Geometry: final body of the model. Coordinates: model frame, mm. Face numbers are marked on the shaded views. A direction names the side the tool comes from. Round coordinates to 2 decimals unless told otherwise and drop trailing zeros. Write each loop counter-clockwise with the first axis right and the second up, starting at its lowest first coordinate (ties: lowest second). Pieces come first, ordered by that corner, then holes.
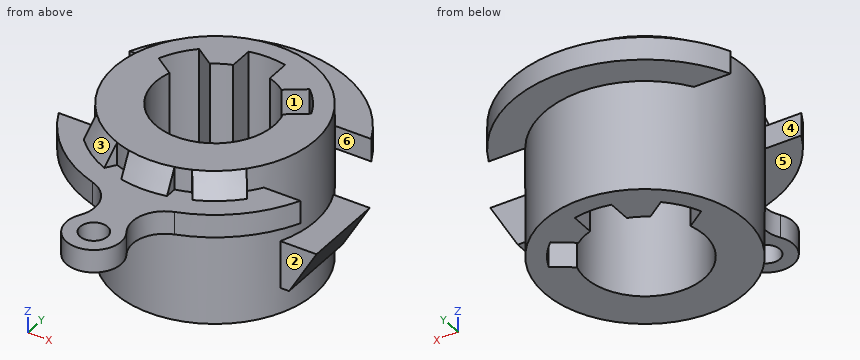
from build123d import *

# Parameters (mm, degrees)
F0_R      = 44
F1_DEPTH  = 34
F3_R      = 6
F4_DEPTH  = 10
F5_W      = 12.3737903833
F5_H      = 20.7846096908
F6_DEPTH  = 18
F4_FACE_R = 6
F8_DEPTH  = 10
F12_DEPTH = 107.2


with BuildPart() as f1:
    # F0 (on Top) → F1 (new body, symmetric)
    with BuildSketch(Plane.XY):
        Circle(F0_R)
        with BuildLine():
            ThreePointArc((-15.6760909215, 20.742713743), (-12.0054639441, 23.0622816626), (-8, 24.7386337537))
            Line((-8, 24.7386337537), (-8, 35.0998575496))
            ThreePointArc((-8, 35.0998575496), (0, 36), (8, 35.0998575496))
            Line((8, 35.0998575496), (8, 24.7386337537))
            ThreePointArc((8, 24.7386337537), (12.0054639441, 23.0622816626), (15.6760909215, 20.742713743))
            Line((15.6760909215, 20.742713743), (24.1635085752, 26.685667564))
            ThreePointArc((24.1635085752, 26.685667564), (29.4894735944, 20.6487517086), (33.3407315568, 13.5792348554))
            Line((33.3407315568, 13.5792348554), (24.8533139031, 7.6362810343))
            ThreePointArc((24.8533139031, 7.6362810343), (0, -26), (-24.8533139031, 7.6362810343))
            Line((-24.8533139031, 7.6362810343), (-33.3407315568, 13.5792348554))
            ThreePointArc((-33.3407315568, 13.5792348554), (-29.4894735944, 20.6487517086), (-24.1635085752, 26.685667564))
            Line((-24.1635085752, 26.685667564), (-15.6760909215, 20.742713743))
        make_face(mode=Mode.SUBTRACT)
    extrude(amount=F1_DEPTH, both=True)

    # F3 (on offset) → F4 (join)
    with BuildSketch(Plane.XY.offset(24)):
        with BuildLine():
            Line((-36.8781778292, -24), (-52.8015151298, -24))
            ThreePointArc((-52.8015151298, -24), (-38.6311115614, -43.2624227191), (-17.8938638331, -55.1707317073))
            ThreePointArc((-17.8938638331, -55.1707317073), (-9.0876412514, -63.6171726174), (-10.252187236, -75.7636022514))
            ThreePointArc((-10.252187236, -75.7636022514), (0, -94), (10.252187236, -75.7636022514))
            ThreePointArc((10.252187236, -75.7636022514), (9.0876412514, -63.6171726174), (17.8938638331, -55.1707317073))
            ThreePointArc((17.8938638331, -55.1707317073), (38.6311115614, -43.2624227191), (52.8015151298, -24))
            Line((52.8015151298, -24), (36.8781778292, -24))
            ThreePointArc((36.8781778292, -24), (0, -44), (-36.8781778292, -24))
        make_face()
        with Locations((0, -82)):
            Circle(F3_R, mode=Mode.SUBTRACT)
        with BuildLine():
            Line((-52.8015151298, 24), (-36.8781778292, 24))
            ThreePointArc((-36.8781778292, 24), (0, 44), (36.8781778292, 24))
            Line((36.8781778292, 24), (52.8015151298, 24))
            ThreePointArc((52.8015151298, 24), (0, 58), (-52.8015151298, 24))
        make_face()
    extrude(amount=-F4_DEPTH)

    # F5 (on Front) → F6 (join, symmetric)
    with BuildSketch(Plane.XZ):
        Polygon((56, -2), (44, -2), (44, -22.7846096908), align=None)
        with Locations((37.8131048083, -12.3923048454)):
            Rectangle(F5_W, F5_H)
    extrude(amount=F6_DEPTH, both=True)

    # F7 (on face) + F4_face (on face) → F8 (join, through all)
    with BuildSketch(Plane.XY.offset(34)):
        with BuildLine():
            ThreePointArc((-16.3854099681, -40.8352585418), (-25.2373631994, -36.0426899487), (-32.7684508539, -29.3637298148))
            Line((-32.7684508539, -29.3637298148), (-35.7052592856, -33.5579269227))
            ThreePointArc((-35.7052592856, -33.5579269227), (-28.1052453812, -40.1384501702), (-19.3222183998, -45.0294556497))
            Line((-19.3222183998, -45.0294556497), (-16.3854099681, -40.8352585418))
        make_face()
        with BuildLine():
            ThreePointArc((10, -42.8485705713), (0, -44), (-10, -42.8485705713))
            Line((-10, -42.8485705713), (-10, -47.9687398208))
            ThreePointArc((-10, -47.9687398208), (0, -49), (10, -47.9687398208))
            Line((10, -47.9687398208), (10, -42.8485705713))
        make_face()
        with BuildLine():
            Line((35.7052592856, -33.5579269227), (32.7684508539, -29.3637298148))
            ThreePointArc((32.7684508539, -29.3637298148), (29.1945327607, -32.9192839668), (25.2373631994, -36.0426899487))
            ThreePointArc((25.2373631994, -36.0426899487), (20.948889946, -38.692945223), (16.3854099681, -40.8352585418))
            Line((16.3854099681, -40.8352585418), (19.3222183998, -45.0294556497))
            ThreePointArc((19.3222183998, -45.0294556497), (28.1052453812, -40.1384501702), (35.7052592856, -33.5579269227))
        make_face()
    with BuildSketch(Plane(origin=(0, -50.9642463073, 24), x_dir=(1, 0, 0), z_dir=(0, 0, 1))):
        with BuildLine():
            ThreePointArc((36.8781778292, 26.9642463073), (0, 6.9642463073), (-36.8781778292, 26.9642463073))
            Line((-36.8781778292, 26.9642463073), (-52.8015151298, 26.9642463073))
            ThreePointArc((-52.8015151298, 26.9642463073), (-38.6311115614, 7.7018235881), (-17.8938638331, -4.2064854001))
            ThreePointArc((-17.8938638331, -4.2064854001), (-9.0876412514, -12.6529263101), (-10.252187236, -24.7993559441))
            ThreePointArc((-10.252187236, -24.7993559441), (0, -43.0357536927), (10.252187236, -24.7993559441))
            ThreePointArc((10.252187236, -24.7993559441), (9.0876412514, -12.6529263101), (17.8938638331, -4.2064854001))
            ThreePointArc((17.8938638331, -4.2064854001), (38.6311115614, 7.7018235881), (52.8015151298, 26.9642463073))
            Line((52.8015151298, 26.9642463073), (36.8781778292, 26.9642463073))
        make_face()
        with Locations((0, -31.0357536927)):
            Circle(F4_FACE_R, mode=Mode.SUBTRACT)
    extrude(amount=-F8_DEPTH)

    # F9 (on Right) → F10 (revolve, cut)
    with BuildSketch(Plane.YZ):
        Polygon((-49, 34), (-49, 24), (-44, 34), align=None)
    revolve(axis=Axis((0, 0, 3.8276161067), (0, 0, 1)), mode=Mode.SUBTRACT)

    # F11 (on face) → F12 (cut)
    with BuildSketch(Plane(origin=(0, 0, -34), x_dir=(1, 0, 0), z_dir=(0, 0, -1))):
        with BuildLine():
            ThreePointArc((24.8533139031, -7.6362810343), (0, 26), (-24.8533139031, -7.6362810343))
            Line((-24.8533139031, -7.6362810343), (-33.3407315568, -13.5792348554))
            ThreePointArc((-33.3407315568, -13.5792348554), (-29.4894735944, -20.6487517086), (-24.1635085752, -26.685667564))
            Line((-24.1635085752, -26.685667564), (-15.6760909215, -20.742713743))
            ThreePointArc((-15.6760909215, -20.742713743), (-12.0054639441, -23.0622816626), (-8, -24.7386337537))
            Line((-8, -24.7386337537), (-8, -35.0998575496))
            ThreePointArc((-8, -35.0998575496), (0, -36), (8, -35.0998575496))
            Line((8, -35.0998575496), (8, -24.7386337537))
            ThreePointArc((8, -24.7386337537), (12.0054639441, -23.0622816626), (15.6760909215, -20.742713743))
            Line((15.6760909215, -20.742713743), (24.1635085752, -26.685667564))
            ThreePointArc((24.1635085752, -26.685667564), (29.4894735944, -20.6487517086), (33.3407315568, -13.5792348554))
            Line((33.3407315568, -13.5792348554), (24.8533139031, -7.6362810343))
        make_face()
    extrude(amount=-F12_DEPTH, mode=Mode.SUBTRACT)


solid = f1.part
1) Section D-D on y = -82. Output: boundary loops of the cut face in (x, z), plus the area to 3 significant figures.
2) First-contact query: P1, Ø2, axis at x = 44, y = 32, coming from the +Z side; P2, Ø17.5, axis at x = 49.5, y = -1.5, coming from the +Z side; P3, Ø8, axis at x = 46, z = -17, coming from the +Y side; P4, Ø10, axis at y = -35, z = -21.5, coming from the -X side. Flat tips, straight axial feed; report the tip coordinate or a pass-through.
3) Section B-B on y = -12. Output: boundary loops of the cut face in (x, z).
4) Line query: probe 1 along Y at (x, z) = (0, 19); probe 2 along X at (y, z) = (21, -10.5); probe 3 along X at (y, z) = (0, 13). Output: solid intervals per line, ascending.
5) Draft query along X for the marked faces 1, 2 and 3. Return one class per face: pulls with the +X half, pulls with the -X half, needs draft (parallel to the pull), parting line crosses it, or undercut.
6) Section C-C on z = -26.5. Output: boundary loops of the cut face in (x, y), plus the area to 3 significant figures.
7) Reachability of the marked faces 4, 5 and 6 from +Z, -Z, +X, -X, +Y, -Y: full face, straight path, thin tool, end or side. Return the list, or none.
8) Section A-A on x = 0. Output: boundary loops of the cut face in (y, z).
Filled in:
1. outline: (-12, 14) - (-6, 14) - (-6, 24) - (-12, 24) - close; (6, 14) - (12, 14) - (12, 24) - (6, 24) - close
1. area: 120 mm2
2. P1: stops at z = 24
2. P2: stops at z = 34
2. P3: stops at y = 18
2. P4: stops at x = -32.19
3. outline: (-42.33, -34) - (-23.07, -34) - (-23.07, 34) - (-42.33, 34) - close; (23.07, -34) - (42.33, -34) - (42.33, -22.78) - (44, -22.78) - (56, -2) - (42.33, -2) - (42.33, 34) - (23.07, 34) - close
4. probe 1: y = -94 to -88, -76 to -26, 36 to 58
4. probe 2: x = -38.67 to -29.24, -16.04 to -15.33, 15.33 to 16.04, 29.24 to 38.67
4. probe 3: x = -44 to -26, 26 to 44
5. face 1: undercut
5. face 2: needs draft
5. face 3: pulls with the -X half
6. outline: circle Ø88 at (0, 0); hole (-33.34, 13.58) - (-24.85, 7.64) arc R26 ccw (long way) to (24.85, 7.64) - (33.34, 13.58) arc R36 ccw to (24.16, 26.69) - (15.68, 20.74) arc R26 ccw to (8, 24.74) - (8, 35.1) arc R36 ccw to (-8, 35.1) - (-8, 24.74) arc R26 ccw to (-15.68, 20.74) - (-24.16, 26.69) arc R36 ccw to start
6. area: 3,470 mm2
7. face 4: +Z, -Z, -X
7. face 5: -Z, -Y
7. face 6: +Z, -Z, +X
8. outline: (-94, 14) - (-88, 14) - (-88, 24) - (-94, 24) - close; (-76, 14) - (-44, 14) - (-44, -34) - (-26, -34) - (-26, 34) - (-44, 34) - (-49, 24) - (-76, 24) - close; (36, -34) - (44, -34) - (44, 14) - (58, 14) - (58, 24) - (44, 24) - (44, 34) - (36, 34) - close
